Here's how the part is built. I have some questions about the finished solid (model axes, mm). A direction names the side the tool comes from. Coordinates: 2 decimals unless noted, no trailing zeros. Write each loop counter-clockwise with the first axis right and the second up, starting at its lowest first coordinate (ties: lowest second). Pieces come first, ordered by that corner, then holes. Notation, with made-up numbers: (33.5, -17) -> (69.5, -17) arc R6 cw to (69.5, -10) -> close; hole circle Ø6 at (-10, 67.5). An arc over 180 degrees is marked (long way). Use a Markdown table: item, result. Add a question column.
Item 1: If I drill on line 1 along X through (y, z) = (4.5, -5.75); line 2 along X through (y, z) = (3.85, -5); line 3 along Z through (x, y) = (-4, 3.3), over which ranges is the centre line in solid material (lowest first)? Write a range as from..to.
Item 2: If we mould it in two halves opening along X, with no side actions, what happens to faces 3 (the flat face through (-4, 0, -3)), 4 (the flat face through (-0.103, 4.437, -2.611)), 5 (the cylindrical face through (-2.81, 4.44, -8.61)), 6 (the cylindrical face through (-5.265, 3.042, -5.806))? For each: pulls with the +X half, pulls with the -X half, needs draft (parallel to the pull), parting line crosses it, or undercut.
Item 3: Imagine slicing it at A-A, the plane x = -8.25. Write out the boundary of the cut face in (y, z).
Item 4: Will these pins go through, and if not, where does the flat tip stop? pin 1 Ø3 at (y, z) = (3.5, -6) entering from +X; pin 2 Ø2.5 at (x, z) = (-4, -5) entering from -Y; pin 3 Ø3 at (y, z) = (1.5, -3) entering from +X.
Item 5: Imagine slicing it at B-B, the plane y = 4.5. Write out the boundary of the cut face in (x, z), and give its area (3 significant figures).
Item 6: Imagine slicing it at C-C, the plane z = -2.75. Write out the boundary of the cut face in (x, y), and give its area (3 significant figures).
Item 7: On a 3-axis mill with a long thin cutter (end or side, diameter ignored), from which of +Z, -Z, +X, -X, +Y, -Y can I reach the whole of each face in a straight line? I mean faces 1 (the flat face through (-4, 6, -5)), 2 (the flat face through (-8, 3, -9.5)). Say none if no direction works.
Item 8: Imagine slicing it at D-D, the plane x = -4. Write out the boundary of the cut face in (y, z), and give its area (3 significant figures).
Autodesk Inventor part; units mm, degrees
ref_plane "YZ Plane" through (0, 0, 0) normal (1, 0, 0) x (0, 1, 0)
ref_plane "XZ Plane" through (0, 0, 0) normal (0, 1, 0) x (-1, 0, 0)
ref_plane "XY Plane" through (0, 0, 0) normal (0, 0, 1) x (1, 0, 0)
sketch "Sketch1" plane through (0, 0, 0) normal (0, 1, 0) x (-1, 0, 0)
  line L0 (0, 0) -> (8, 0)
  line L1 (8, 0) -> (7.7971, -5.1496)
  line L2 (0.2029, -5.1496) -> (0, 0)
  arc A0 (0.2029, -5.1496) -> (7.7971, -5.1496) centre (4, -5) ccw
  line L3 (4, -5) -> (4, -1.2)
  dimension "d0" = 3.8
  dimension "d1" = 5
  dimension "d2" = 8
extrude "Extrusion1" add sketch "Sketch1" along normal blind 9
sketch "Sketch2" plane through (-8, 0, 0) normal (0, 0, 1) x (1, 0, 0)
  line L0 (8, 0) -> (0, 0)
  line L1 (0, 0) -> (0, 9)
  circle A0 centre (-0.25, 4.5) radius 4
  line L2 (4, 0) -> (4, -1.6223)
  point P0 (0, 4.5)
  dimension "d5" = 8
  dimension "d6" = 4.25
extrude "Extrusion2" add sketch "Sketch2" against normal blind 9.5
hole "Hole2" at (-8.25, 4.5, -9.5) direction (0, 0, 1) diameter 2.459 depth 12.05
hole "Hole3" at (-4, 0, -5) direction (0, 1, 0) diameter 3 depth 6
properties part number "500-172" material "ABS Plastic"
Ans:
| question | item | result |
|---|---|---|
| 1 | line 1 | x = -12.25..-9.48, -7.02..-5.3, -2.7..-0.27 |
| 1 | line 2 | x = -12.2..-9.29, -7.21..-5.5, -2.5..-0.2 |
| 1 | line 3 | z = -8.8..-6.5, -3.5..0 |
| 2 | face 3 | needs draft |
| 2 | face 4 | pulls with the +X half |
| 2 | face 5 | undercut |
| 2 | face 6 | undercut |
| 3 | outline | (0.5, -9.5) -> (3.27, -9.5) -> (3.27, 0) -> (0.5, 0) -> close; (5.73, -9.5) -> (8.5, -9.5) -> (8.5, 0) -> (5.73, 0) -> close |
| 4 | pin 1 | stops at x = -0.18 |
| 4 | pin 2 | stops at y = 6 |
| 4 | pin 3 | stops at x = -0.06 |
| 5 | outline | (-12.25, -9.5) -> (-9.48, -9.5) -> (-9.48, 0) -> (-12.25, 0) -> close; (-7.02, -9.5) -> (-4.25, -9.5) -> (-4.25, -8.79) arc R3.8 ccw to (-0.2, -5.15) -> (0, 0) -> (-7.02, 0) -> close; hole circle Ø3 at (-4, -5) |
| 5 | area | 78.6 mm^2 |
| 6 | outline | (-7.89, 0) -> (-0.11, 0) -> (-0.11, 9) -> (-7.89, 9) -> (-7.89, 8.48) arc R4 ccw (long way) to (-7.89, 0.52) -> close; hole circle Ø2.46 at (-8.25, 4.5) |
| 6 | area | 93.3 mm^2 |
| 7 | face 1 | -Y |
| 7 | face 2 | -Z, +X, -X, +Y, -Y |
| 8 | outline | (0, -8.8) -> (9, -8.8) -> (9, 0) -> (0, 0) -> (0, -3.5) -> (6, -3.5) -> (6, -6.5) -> (0, -6.5) -> close |
| 8 | area | 61.2 mm^2 |
